Part model, mm, in its own coordinate system. A direction names the side the tool comes from. Round coordinates to 2 decimals unless told otherwise and drop trailing zeros. Loops run counter-clockwise (first coordinate to the right, second up) from the corner with the lowest first, then second, coordinate; pieces in that order, holes last.
from build123d import *

# Parameters (mm, degrees)
BOSS_EXTRUDE1_DEPTH = 3
BOSS_EXTRUDE2_DEPTH = 25
BOSS_EXTRUDE3_START = -3
BOSS_EXTRUDE3_DEPTH = 13
BOSS_EXTRUDE5_DEPTH = 28
CUT_EXTRUDE9_START  = -4.767335
CUT_EXTRUDE9_DEPTH  = 4.767335
CUT_EXTRUDE10_DEPTH = 3
CUT_EXTRUDE11_DEPTH = 3
CUT_EXTRUDE14_START = -13
CUT_EXTRUDE14_DEPTH = 11.360991
CUT_EXTRUDE15_START = -13
CUT_EXTRUDE15_DEPTH = 11.360991
CHAMFER4_SIZE       = 1


with BuildPart() as part:
    # Sketch12 → Boss-Extrude1 (new body)
    with BuildSketch(Plane(origin=(0, 0, 0), x_dir=(1, 0, 0), z_dir=(0, 1, 0))):
        Polygon((-27, -6.414360409), (-27, -2.352653961), (-25, -2), (25, -2), (27, -2.352653961), (27, -6.414360409), (35.023054857, -7.829041448), (35.023054857, -1.736481777), (25.174977327, 0), (-25.174977327, 0), (-35.023054857, -1.736481777), (-35.023054857, -7.829041448), align=None)
    extrude(amount=BOSS_EXTRUDE1_DEPTH)

    # Sketch13 → Boss-Extrude2 (add)
    with BuildSketch(Plane.XZ):
        Polygon((25.174977327, 0), (35.023054857, 1.736481777), (35.023054857, 3.767335), (27, 2.352653961), (25, 2), (-25, 2), (-27, 2.352653961), (-35.023054857, 3.767335), (-35.023054857, 1.736481777), (-25.174977327, 0), align=None)
    extrude(amount=BOSS_EXTRUDE2_DEPTH)

    # Sketch14 → Boss-Extrude3 (add)
    with BuildSketch(Plane.XZ.offset(BOSS_EXTRUDE3_START)):
        Polygon((-35.023054857, 5.798188224), (-27, 4.383507185), (-27, 7.429787021), (-35.023054857, 8.84446806), align=None)
        Polygon((27, 7.429787021), (35.023054857, 8.84446806), (35.023054857, 5.798188224), (27, 4.383507185), align=None)
    extrude(amount=BOSS_EXTRUDE3_DEPTH)

    # Sketch24 → Boss-Extrude5 (add)
    with BuildSketch(Plane(origin=(0, 3, 0), x_dir=(1, 0, 0), z_dir=(0, 1, 0))):
        Polygon((-35.023054857, -0.721055165), (-25.262465991, 1), (25.262465991, 1), (35.023054857, -0.721055165), (35.023054857, -1.736481777), (25.174977327, 0), (-25.174977327, 0), (-35.023054857, -1.736481777), align=None)
    extrude(amount=-BOSS_EXTRUDE5_DEPTH)

    # Sketch26 → Cut-Extrude9 (cut)
    with BuildSketch(Plane(origin=(0, 0, -1), x_dir=(-1, 0, 0), z_dir=(0, 0, -1)).offset(CUT_EXTRUDE9_START)):
        Polygon((-25.262465991, -25), (-35.023054857, -25), (-35.023054857, -15.239411133), align=None)
        Polygon((25.262465991, -25), (35.023054857, -15.239411133), (35.023054857, -25), align=None)
    extrude(amount=CUT_EXTRUDE9_DEPTH, mode=Mode.SUBTRACT)

    # Sketch27 → Cut-Extrude10 (cut)
    with BuildSketch(Plane(origin=(0.456418791, 0, 2.588479594), x_dir=(0.9848077530121054, 0, -0.17364817766751295), z_dir=(0.17364817766751295, 0, 0.9848077530121054))):
        Polygon((-36.026801719, -3.5), (-31.953390013, -10), (-36.026801719, -10), align=None)
    extrude(amount=-CUT_EXTRUDE10_DEPTH, mode=Mode.SUBTRACT)

    # Sketch28 → Cut-Extrude11 (cut)
    with BuildSketch(Plane(origin=(-0.456418791, 0, 2.588479594), x_dir=(0.9848077530121067, 0, 0.17364817766750618), z_dir=(-0.17364817766750618, 0, 0.9848077530121067))):
        Polygon((36.026801719, -3.5), (31.953390013, -10), (36.026801719, -10), align=None)
    extrude(amount=-CUT_EXTRUDE11_DEPTH, mode=Mode.SUBTRACT)

    # Sketch31 → Cut-Extrude14 (cut)
    with BuildSketch(Plane.XZ.offset(10).offset(CUT_EXTRUDE14_START)):
        Polygon((35.023054857, 5.798188224), (32.023054857, 8.315487118), (35.023054857, 8.84446806), align=None)
    extrude(amount=CUT_EXTRUDE14_DEPTH, mode=Mode.SUBTRACT)

    # Sketch33 → Cut-Extrude15 (cut)
    with BuildSketch(Plane.XZ.offset(10).offset(CUT_EXTRUDE15_START)):
        Polygon((-35.023054857, 5.798188224), (-32.023054857, 8.315487118), (-35.023054857, 8.84446806), align=None)
    extrude(amount=CUT_EXTRUDE15_DEPTH, mode=Mode.SUBTRACT)

    # Chamfer4
    chamfer4_edges = [part.edges().sort_by_distance(p)[0] for p in [
        (35.023054857, 3, 3.259621695),
        (-35.023054857, 3, 3.259621695),
    ]]
    chamfer(chamfer4_edges, length=CHAMFER4_SIZE)


solid = part.part
1) Drop flat-ended pins along their axis: pin 1 Ø4 at (x, z) = (-30.5, 3) entering from -Y; pin 2 Ø1.1 at (x, z) = (30, 6) entering from -Y; pin 3 Ø4 at (x, z) = (32.5, 3.5) entering from -Y. Give the stop position or say it passes through.
Values:
pin 1: stops at y = -21.73
pin 2: stops at y = -10
pin 3: stops at y = -19.69
2) Slice it at B-B, the plane y = -5.5. Give the cut face in (x, z).
Values:
outline: (-35.02, 0.72) - (-25.26, -1) - (25.26, -1) - (35.02, 0.72) - (35.02, 3.77) - (25, 2) - (-25, 2) - (-35.02, 3.77) - close; (-34.31, 5.67) - (-27, 4.38) - (-27, 7.43) - (-32.02, 8.32) - (-34.16, 6.52) - close; (27, 4.38) - (34.31, 5.67) - (34.16, 6.52) - (32.02, 8.32) - (27, 7.43) - close
3) Slice it at D-D, the plane y = 1.25. Give the cut face in (x, z).
Values:
outline: (-35.02, 0.72) - (-25.26, -1) - (25.26, -1) - (35.02, 0.72) - (35.02, 5.8) - (32.02, 8.32) - (27, 7.43) - (27, 2.35) - (25, 2) - (-25, 2) - (-27, 2.35) - (-27, 7.43) - (-32.02, 8.32) - (-35.02, 5.8) - close
4) Wall check: line 1 along X through (y, z) = (1.75, 3.5); line 2 along Z through (x, y) = (10, -12); line 3 along X through (y, z) = (-3.5, 7.25). Give the ranges that are in metal, low to high.
Values:
line 1: x = -35.02 to -27, 27 to 35.02
line 2: z = -1 to 2
line 3: x = -33.29 to -27, 27 to 33.29
5) Slice it at C-C, the plane x = -8. Give the cut face in (y, z), then the cut area to 3 significant figures.
Values:
outline: (-25, -1) - (3, -1) - (3, 2) - (-25, 2) - close
area: 84.0 mm2
6) Mould opens along X. For faces 6 (the face through (-29, -10, 6)), 7 (the face through (29.476, -3.409, 7.866)), 8 (the face through (-29.476, -3.409, 7.866)), 9 (the face through (32.71, -7.76, 6.6)) say: released by +X, released by -X, zero draft, split by the parting line, or undercut.
Values:
face 6: zero draft
face 7: undercut
face 8: undercut
face 9: released by +X
7) Slice it at A-A, the plane y = -12.75. Give the cut face in (x, z), then the cut area to 3 significant figures.
Values:
outline: (-35.02, 0.72) - (-25.26, -1) - (25.26, -1) - (35.02, 0.72) - (35.02, 3.77) - (25, 2) - (-25, 2) - (-35.02, 3.77) - close
area: 211 mm2
8) Tool access for faces 1 (the face through (-31.07, -4.93, 5.1)), 2 (the face through (27, -2, 5)), 3 (the face through (29, -10, 6)), 4 (the face through (0, -25, 1)), 5 (the face through (31, 0, 4)): list every direction of +Z, -Z, +X, -X, +Y, -Y with a clear straight run to the whole face (end or side of a thin tool).
Values:
face 1: -X, -Y
face 2: +Z, +Y, -Y
face 3: +Z, +X, -X, -Y
face 4: +Z, -Z, +X, -X, -Y
face 5: -Y
